Check sheet for the modelled part. Datum: model origin and axes. Units: mm. A direction names the side the tool comes from. Give positions to 0.01 mm unless a question says otherwise; leave off trailing zeros. Write each loop counter-clockwise with the first axis right and the second up, starting at its lowest first coordinate (ties: lowest second). Pieces come first, ordered by that corner, then holes. Notation, with made-up numbers: (-20, -18) -> (5, -18) arc R18 cw to (5, -4) -> close; hole circle Ø6 at (38.25, -2.75). An arc over 180 degrees is marked (long way). Return JSON: item names as keys, results as strings.
from build123d import *

# Parameters (mm, degrees)
SKETCH1_R           = 7
BOSS_EXTRUDE1_DEPTH = 7
SKETCH2_R           = 2.7
CUT_EXTRUDE2_DEPTH  = 10
SKETCH3_R           = 8
SKETCH3_W           = 5.4
SKETCH3_H           = 8.674169728
BOSS_EXTRUDE2_DEPTH = 1
SKETCH4_R           = 8
CUT_EXTRUDE3_DEPTH  = 0.5
SKETCH5_R           = 7.1
SKETCH5_W           = 5.4
SKETCH5_H           = 8.674169728
BOSS_EXTRUDE3_DEPTH = 6
SKETCH6_R           = 5.108845772
CUT_EXTRUDE4_DEPTH  = 1.1
CUT_EXTRUDE5_DEPTH  = 10.1
SKETCH9_R           = 5.298635414
CUT_EXTRUDE6_DEPTH  = 1.6
CUT_EXTRUDE7_DEPTH  = 10.6


with BuildPart() as part:
    # Sketch1 → Boss-Extrude1 (new body)
    with BuildSketch(Plane(origin=(0, 0, 0), x_dir=(1, 0, 0), z_dir=(0, 1, 0))):
        with Locations(Location((0, 0, 0), (0, 0, 270))):
            Circle(SKETCH1_R)
    extrude(amount=BOSS_EXTRUDE1_DEPTH)

    # Sketch2 → Cut-Extrude2 (cut)
    with BuildSketch(Plane.XZ):
        with BuildLine():
            Line((2.7, 4.337084864), (-2.7, 4.337084864))
            Line((-2.7, 4.337084864), (-2.7, 0))
            ThreePointArc((-2.7, 0), (0, 2.7), (2.7, 0))
            Line((2.7, 0), (2.7, 4.337084864))
        make_face()
        with BuildLine():
            ThreePointArc((2.7, 0), (0, -2.7), (-2.7, 0))
            Line((-2.7, 0), (-2.7, -4.337084864))
            Line((-2.7, -4.337084864), (2.7, -4.337084864))
            Line((2.7, -4.337084864), (2.7, 0))
        make_face()
        Circle(SKETCH2_R)
    extrude(amount=-CUT_EXTRUDE2_DEPTH, mode=Mode.SUBTRACT)

    # Sketch3 → Boss-Extrude2 (add)
    with BuildSketch(Plane.XZ):
        with Locations(Location((0, 0, 0), (0, 0, 270))):
            Circle(SKETCH3_R)
        Rectangle(SKETCH3_W, SKETCH3_H, mode=Mode.SUBTRACT)
    extrude(amount=-BOSS_EXTRUDE2_DEPTH)

    # Sketch4 → Cut-Extrude3 (cut)
    with BuildSketch(Plane.XZ):
        with Locations(Location((0, 0, 0), (0, 0, 270))):
            Circle(SKETCH4_R)
    extrude(amount=-CUT_EXTRUDE3_DEPTH, mode=Mode.SUBTRACT)

    # Sketch5 → Boss-Extrude3 (add)
    with BuildSketch(Plane(origin=(0, 7, 0), x_dir=(1, 0, 0), z_dir=(0, 1, 0))):
        with Locations(Location((0, 0, 0), (0, 0, 270))):
            Circle(SKETCH5_R)
        Rectangle(SKETCH5_W, SKETCH5_H, mode=Mode.SUBTRACT)
    extrude(amount=-BOSS_EXTRUDE3_DEPTH)

    # Sketch6 → Cut-Extrude4 (cut)
    with BuildSketch(Plane.XZ.offset(-0.5)):
        with Locations(Location((0, 0, 0), (0, 0, 270))):
            Circle(SKETCH6_R)
    extrude(amount=-CUT_EXTRUDE4_DEPTH, mode=Mode.SUBTRACT)

    # Sketch8 → Cut-Extrude5 (cut)
    with BuildSketch(Plane.XZ.offset(-1.6)):
        with BuildLine():
            Line((-2.7, 4.337084864), (2.7, 4.337084864))
            ThreePointArc((2.7, 4.337084864), (0, 5.108845772), (-2.7, 4.337084864))
        make_face()
        with BuildLine():
            Line((2.7, -4.337084864), (-2.7, -4.337084864))
            ThreePointArc((-2.7, -4.337084864), (0, -5.108845772), (2.7, -4.337084864))
        make_face()
    extrude(amount=-CUT_EXTRUDE5_DEPTH, mode=Mode.SUBTRACT)

    # Sketch9 → Cut-Extrude6 (cut)
    with BuildSketch(Plane.XZ.offset(-0.5)):
        with Locations(Location((0, 0, 0), (0, 0, 270))):
            Circle(SKETCH9_R)
    extrude(amount=-CUT_EXTRUDE6_DEPTH, mode=Mode.SUBTRACT)

    # Sketch10 → Cut-Extrude7 (cut)
    with BuildSketch(Plane.XZ.offset(-2.1)):
        with BuildLine():
            Line((-2.7, -4.337084864), (-2.7, -4.55911584))
            ThreePointArc((-2.7, -4.55911584), (0, -5.298635414), (2.7, -4.55911584))
            Line((2.7, -4.55911584), (2.7, -4.337084864))
            ThreePointArc((2.7, -4.337084864), (0, -5.108845772), (-2.7, -4.337084864))
        make_face()
        with BuildLine():
            Line((-2.7, 4.55911584), (-2.7, 4.337084864))
            ThreePointArc((-2.7, 4.337084864), (0, 5.108845772), (2.7, 4.337084864))
            Line((2.7, 4.337084864), (2.7, 4.55911584))
            ThreePointArc((2.7, 4.55911584), (0, 5.298635414), (-2.7, 4.55911584))
        make_face()
    extrude(amount=-CUT_EXTRUDE7_DEPTH, mode=Mode.SUBTRACT)


solid = part.part
(1) Set-up check for faces 4 (the cylindrical face through (5.987, 4.042, 3.817)), 5 (the flat face through (-4, 2.1, 0)), 6 (the flat face through (2.7, 5, 0)): record each of +Z, -Z, +X, -X, +Y, -Y from which the full face is reachable in a straight line by a thin tool's end or side.
Reply:
{"face 4": "+Y", "face 5": "-Y", "face 6": "+Y, -Y"}
(2) Depth check by flat-ended pin: pin 1 Ø2 at (x, z) = (-4, -0.5) entering from -Y; pin 2 Ø1.5 at (y, z) = (5.5, 1.5) entering from +X; pin 3 Ø2 at (y, z) = (5, 4) entering from -X. Enter the tip coordinate at first touch or a pass-through.
Reply:
{"pin 1": "y = 2.1", "pin 2": "x = 7.06", "pin 3": "x = -6.44"}
(3) Cross-section at B-B on y = 4.5. Enter the section's corners in (x, z).
Reply:
{"outline": "circle Ø14.2 at (0, 0); hole (-2.7, -4.56) arc R5.3 ccw to (2.7, -4.56) -> (2.7, 4.56) arc R5.3 ccw to (-2.7, 4.56) -> close"}
(4) Release check for a two-part mould opening along X. For faces 1 (the cylindrical face through (-7.81, 0.75, 1.73)), 2 (the flat face through (-2.7, 5, 0)), 3 (the flat face through (-1.7, 0.5, -5.2)) record: pulls with the +X half, pulls with the -X half, needs draft (parallel to the pull), parting line crosses it, or undercut.
Reply:
{"face 1": "parting line crosses it", "face 2": "undercut", "face 3": "needs draft"}
(5) Cross-section at D-D on z = 2.5. Enter the section's corners in (x, y).
Reply:
{"outline": "(-7.6, 0.5) -> (-4.67, 0.5) -> (-4.67, 2.1) -> (-2.7, 2.1) -> (-2.7, 7) -> (-6.65, 7) -> (-6.65, 1) -> (-7.6, 1) -> close; (2.7, 2.1) -> (4.67, 2.1) -> (4.67, 0.5) -> (7.6, 0.5) -> (7.6, 1) -> (6.65, 1) -> (6.65, 7) -> (2.7, 7) -> close"}
(6) Cross-section at A-A on z = 0. Enter the section's corners in (x, y).
Reply:
{"outline": "(-8, 0.5) -> (-5.3, 0.5) -> (-5.3, 2.1) -> (-2.7, 2.1) -> (-2.7, 7) -> (-7.1, 7) -> (-7.1, 1) -> (-8, 1) -> close; (2.7, 2.1) -> (5.3, 2.1) -> (5.3, 0.5) -> (8, 0.5) -> (8, 1) -> (7.1, 1) -> (7.1, 7) -> (2.7, 7) -> close"}
(7) Thickness scan on L1, parallel to X at y = 2.5, z = 0; L2, parallel to Y at x = -0.5, z = 7.75; L3, parallel to Y at x = -3, z = 1. Record the ranges inside material, lowest first.
Reply:
{"L1": "-7.1 to -2.7, 2.7 to 7.1", "L2": "0.5 to 1", "L3": "2.1 to 7"}
